Could you check a few things on this model? Use its own coordinates, in mm. A direction names the side the tool comes from. Coordinates: 2 decimals unless noted, no trailing zeros. Order: outer loops, then holes, each group sorted by start corner. A loop starts at its lowest first (then second) coordinate and runs counter-clockwise, first axis right, second up. Notation, with made-up numbers: (22, -39) - (60, -39) arc R19 cw to (60, -12) - close; hole circle Ø2 at (-25.5, 10). An arc over 180 degrees is marked (long way). One line per item, written item: value.
from build123d import *

# Parameters (mm, degrees)
F0_W     = 220
F0_H     = 220
F0_R     = 3.5
F1_DEPTH = 5
F2_R     = 3.75
F3_DEPTH = 5.001
F4_R     = 6
F5_DEPTH = 3


with BuildPart() as f1:
    # F0 (on Top) → F1 (new body)
    with BuildSketch(Plane.XY):
        Rectangle(F0_W, F0_H)
        with Locations((-100, -100)):
            Circle(F0_R, mode=Mode.SUBTRACT)
        with Locations((100, -100)):
            Circle(F0_R, mode=Mode.SUBTRACT)
        with Locations((-100, 100)):
            Circle(F0_R, mode=Mode.SUBTRACT)
        with Locations((100, 100)):
            Circle(F0_R, mode=Mode.SUBTRACT)
    extrude(amount=F1_DEPTH)

    # F2 (on face) → F3 (cut, through all)
    with BuildSketch(Plane.XY.offset(5)):
        with Locations((-56, 7.5)):
            Circle(F2_R)
        with Locations((78, 74.5)):
            Circle(F2_R)
        with Locations((78, -59)):
            Circle(F2_R)
    extrude(amount=-F3_DEPTH, mode=Mode.SUBTRACT)

    # F4 (on face) → F5 (cut)
    with BuildSketch(Plane.XY.offset(5)):
        with Locations((-56, 7.5)):
            Circle(F4_R)
        with Locations((78, 74.5)):
            Circle(F4_R)
        with Locations((78, -59)):
            Circle(F4_R)
    extrude(amount=-F5_DEPTH, mode=Mode.SUBTRACT)


solid = f1.part
Item 1: I'm going to push flat-ended pins straight in: pin 1 Ø9.5 at (x, y) = (-56, 7.5) entering from -Z; pin 2 Ø5.5 at (x, y) = (-100, -100) entering from -Z; pin 3 Ø10 at (x, y) = (-56, 7.5) entering from +Z. Where does each tip first touch, or does it pass through?
Conclusion:
pin 1: z = 0
pin 2: through
pin 3: z = 2
Item 2: I want a section at D-D on y = -100. Please give me the cut outline in (x, z), then the cut area to 3 significant figures.
Conclusion:
outline: (-110, 0) - (-103.5, 0) - (-103.5, 5) - (-110, 5) - close; (-96.5, 0) - (96.5, 0) - (96.5, 5) - (-96.5, 5) - close; (103.5, 0) - (110, 0) - (110, 5) - (103.5, 5) - close
area: 1,030 mm²
Item 3: Thinking about a two-plate mould opening in Y: for faces 1 (the face through (-2, 110, 2)), 2 (the face through (81.577, 75.626, 1.014)), 3 (the face through (-2, 2, 5)), 4 (the face through (-61.994, 7.764, 3.521)), which applies, pulls with the +Y half, pulls with the -Y half, needs draft (parallel to the pull), parting line crosses it, or undercut?
Conclusion:
face 1: pulls with the +Y half
face 2: undercut
face 3: needs draft
face 4: undercut
Item 4: If I drill on probe 1 along Y at (x, z) = (-100, 1.1); probe 2 along Y at (x, z) = (78, 2.85); probe 3 along Y at (x, z) = (-56, 3.55), over which ranges is the centre line in solid material (lowest first)?
Conclusion:
probe 1: -110 to -103.5, -96.5 to 96.5, 103.5 to 110
probe 2: -110 to -65, -53 to 68.5, 80.5 to 110
probe 3: -110 to 1.5, 13.5 to 110
Item 5: I want a section at C-C on x = 78. Please give me the cut outline in (y, z), then the cut area to 3 significant figures.
Conclusion:
outline: (-110, 0) - (-62.75, 0) - (-62.75, 2) - (-65, 2) - (-65, 5) - (-110, 5) - close; (-55.25, 0) - (70.75, 0) - (70.75, 2) - (68.5, 2) - (68.5, 5) - (-53, 5) - (-53, 2) - (-55.25, 2) - close; (78.25, 0) - (110, 0) - (110, 5) - (80.5, 5) - (80.5, 2) - (78.25, 2) - close
area: 998 mm²
Item 6: For faces 5 (the face through (73.58, 78.56, 3.52)), 6 (the face through (103.233, 98.659, 2.465)), which set-ups out of +Z, -Z, +X, -X, +Y, -Y let a thin tool reach every point of the face, with its end or its side?
Conclusion:
face 5: +Z
face 6: +Z, -Z
Item 7: I want a section at A-A on x = -56. Please give me the cut outline in (y, z).
Conclusion:
outline: (-110, 0) - (3.75, 0) - (3.75, 2) - (1.5, 2) - (1.5, 5) - (-110, 5) - close; (11.25, 0) - (110, 0) - (110, 5) - (13.5, 5) - (13.5, 2) - (11.25, 2) - close
Item 8: I want a section at B-B on y = 74.5. Please give me the cut outline in (x, z), then the cut area to 3 significant figures.
Conclusion:
outline: (-110, 0) - (74.25, 0) - (74.25, 2) - (72, 2) - (72, 5) - (-110, 5) - close; (81.75, 0) - (110, 0) - (110, 5) - (84, 5) - (84, 2) - (81.75, 2) - close
area: 1,050 mm²
